Autodesk Inventor part; units mm, degrees
ref_plane "YZ Plane" through (0, 0, 0) normal (1, 0, 0) x (0, 1, 0)
ref_plane "XZ Plane" through (0, 0, 0) normal (0, 1, 0) x (-1, 0, 0)
ref_plane "XY Plane" through (0, 0, 0) normal (0, 0, 1) x (1, 0, 0)
sketch "Skizze1" plane through (0, 0, 0) normal (0, 0, 1) x (1, 0, 0)
  line L0 (45, 140.75) -> (-45, 140.75)
  line L1 (-45, 140.75) -> (-45, -140.75)
  line L2 (-45, -140.75) -> (45, -140.75)
  line L3 (45, -140.75) -> (45, 140.75)
  line L4 (0, 197.05) -> (0, -197.05)
  line L5 (-63, 0) -> (63, 0)
  point P0 (0, 0)
  point P1 (45, 0)
  point P2 (0, -140.75)
  dimension "d0" = 281.5
  dimension "d1" = 90
extrude "Extrusion1" add sketch "Skizze1" along normal blind 8
sketch "Skizze2" plane through (-45, -140.75, 0) normal (0, -1, 0) x (1, 0, 0)
  line L0 (90, 8) -> (0, 8)
  line L1 (86.8, 8) -> (88, 8)
  line L2 (88, 8) -> (88, 5.5)
  line L3 (88, 5.5) -> (86.8, 5.5)
  line L4 (86.8, 5.5) -> (86.8, 8)
  line L5 (90, 0) -> (90, 8)
  point P0 (45, 0)
  dimension "d4" = 1.2
  dimension "d5" = 2.5
  dimension "d8" = 2
extrude "Extrusion2" cut sketch "Skizze2" against normal through all
sketch "Skizze3" plane through (0, 0, 0) normal (0, 0, -1) x (-1, 0, 0)
  line L0 (-45, -140.75) -> (-41, -140.75)
  line L1 (-41, -140.75) -> (-41, 39.25)
  line L2 (-41, 39.25) -> (-45, 39.25)
  line L3 (-45, 39.25) -> (-45, -140.75)
  point P0 (0, 0)
  dimension "d9" = 4
  dimension "d10" = 180
extrude "Extrusion3" cut sketch "Skizze3" against normal through all
sketch "Skizze4" plane through (0, 0, 0) normal (0, 0, -1) x (-1, 0, 0)
  line L0 (-41, 39.25) -> (-43, 39.25)
  line L1 (-43, 39.25) -> (-43, 35.25)
  line L2 (-43, 35.25) -> (-41, 35.25)
  line L3 (-41, 35.25) -> (-41, 39.25)
  point P0 (0, 0)
  dimension "d13" = 4
  dimension "d14" = 2
extrude "Extrusion4" add sketch "Skizze4" against normal blind 5.5
sketch "Skizze5" plane through (41.8, 39.25, 5.5) normal (0, 0, 1) x (1, 0, 0)
  line L0 (0, 0) -> (-0.8, 0)
  line L1 (-0.8, 0) -> (-0.8, -4)
  line L2 (-0.8, -4) -> (0, -4)
  line L3 (0, -4) -> (0, 0)
  point P0 (-41.8, -39.25)
extrude "Extrusion5" add sketch "Skizze5" along normal up to surface (2.5 mm away)
sketch "Skizze6" plane through (-45, -140.75, 0) normal (-1, 0, 0) x (0, 0, 1)
  line L0 (0, 0) -> (8, 0)
  line L1 (0, 281.5) -> (8, 281.5)
  line L2 (0, 281.5) -> (0, 0)
  point P0 (0, 140.75)
  point P1 (4, 60)
  point P2 (4, 229.5)
  dimension "d19" = 60
  dimension "d41" = 52
  dimension "d42" = 4
hole "Bohrung1" at (-45, -80.75, 4) at (-45, 88.75, 4) direction (1, 0, 0) diameter 2.459 depth 12 tip angle 118
sketch "Skizze7" plane through (-45, 140.75, 0) normal (0, 1, 0) x (1, 0, 0)
  arc A0 (90, -95.2303) -> (67.5, -77) centre (67.5, -100) ccw
  line L0 (90, 0) -> (90, -95.2303)
  line L1 (0, 0) -> (90, 0)
  line L2 (0, -77) -> (0, 0)
  line L3 (0, -77) -> (67.5, -77)
  point P0 (22, -4)
  point P1 (68, -4)
hole "Bohrung2" at (-23, 140.75, 4) at (23, 140.75, 4) direction (0, -1, 0) diameter 2.459 depth 10 tip angle 118
sketch "Skizze8" plane through (0, 0, 0) normal (0, 0, -1) x (-1, 0, 0)
  line L0 (-41.8, 35.25) -> (-41.8, 140.75)
  line L1 (45, 140.75) -> (-41.8, 140.75)
  line L2 (45, -140.75) -> (45, 140.75)
  line L3 (-41, -140.75) -> (45, -140.75)
  line L4 (-41, -140.75) -> (-41, 35.25)
  line L5 (-41.8, 35.25) -> (-41, 35.25)
  circle A0 centre (-23, -136.75) radius 3.1
  circle A1 centre (23, -136.75) radius 3.1
  line L6 (45, -140.75) -> (45, 140.75)
  line L7 (-41, -140.75) -> (45, -140.75)
  line L8 (-41, 140.75) -> (-41, -140.75)
  line L9 (45, 140.75) -> (-41, 140.75)
  point P0 (0, 0)
hole "Bohrung3" at (23, -136.75, 0) at (-23, -136.75, 0) direction (0, 0, 1) diameter 3.2 end through all countersink diameter 6.2 countersink angle 90
sketch "Skizze10" plane through (41, -140.75, 8) normal (1, 0, 0) x (0, 0, -1)
  circle A0 centre (4, 155) radius 3.1
  circle A1 centre (4, 60) radius 3.1
  point P0 (8, 140.75)
hole "Bohrung4" at (41, -80.75, 4) at (41, 14.25, 4) direction (-1, 0, 0) diameter 2.459 depth 10 tip angle 118
properties part number "Wand2" material "Polycarbonate, Smoke"
Here's how the part is built. I have some questions about the finished solid (model axes, mm). A direction names the side the tool comes from. Round coordinates to 2 decimals unless told otherwise and drop trailing zeros. Loops run counter-clockwise (first coordinate to the right, second up) from the corner with the lowest first, then second, coordinate; pieces in that order, holes last. Notation, with made-up numbers: (28, 38.25) - (78, 38.25) arc R19 ccw to (78, 52.25) - close; hole circle Ø5 at (0, 56.25). An arc over 180 degrees is marked (long way). One line per question, with ' | ' between items. Start each with the question number.
Q1. For faces 1 (the flat face through (1, 140.75, 4)), 2 (the flat face through (41, -54, 4)), which set-ups out of +Z, -Z, +X, -X, +Y, -Y let a thin tool reach every point of the face, with its end or its side?
Q2. Will these pins go through, and if not, where does the flat tip stop? pin 1 (3 mm diameter, centred on y = -80.75, z = 4, fed in from -X); pin 2 (4 mm diameter, centred on y = 14.25, z = 4, fed in from +X); pin 3 (2 mm diameter, centred on y = 38, z = 3, fed in from +X).
Q3. I want a section at A-A (y = -1.5). Write out the boundary of the cut face in (x, z), then the cut area to 3 significant figures.
Q4. Please list where these lines run through material, in increasing order: line 1 (X direction, y = 138.75, z = 4); line 2 (X direction, y = -136.75, z = 6.25); line 3 (Y direction, x = -40.5, z = 4.75). Write a range as [from, to].
Response values:
1) face 1: +Z, -Z, +X, -X, +Y | face 2: +Z, -Z, +X, -Y
2) pin 1: stops at x = -45 | pin 2: stops at x = 41 | pin 3: stops at x = 43
3) outline: (-45, 0) - (41, 0) - (41, 8) - (-45, 8) - close | area: 688 mm²
4) line 1: x = [-45, -24.23], [-21.77, 21.77], [24.23, 45] | line 2: x = [-45, -24.6], [-21.4, 21.4], [24.6, 41] | line 3: y = [-140.75, -81.72], [-79.78, 87.78], [89.72, 140.75]
